Source: CAD feature listing. Evaluate the final solid. Frame: model axes, mm. Face numbers are marked on the shaded views. A direction names the side the tool comes from. Give positions to 0.01 mm unless a question says otherwise; leave off trailing zeros. Order: outer loops, then holes, each group sorted by start corner. A loop starts at its lowest first (then second) coordinate and runs counter-clockwise, first axis right, second up. Notation, with made-up numbers: (65, 34.5) - (106, 34.5) arc R14 ccw to (106, 48.5) - close; hole circle Ø11 at (51, 83). An arc over 180 degrees is marked (long way). Write each question's results on one line, items separated by ' | '. Start each with the question number.
Item 1: Section C-C on y = 1912.5. Output: boundary loops of the cut face in (x, z), and give its area (3 significant figures).
Item 2: Mould query, pull axis X, two halves, no side actions, for the marked faces 1, 2 and 3. Classes: released by +X, released by -X, zero draft, split by the parting line, or undercut.
Item 3: Contact query for flat-ended pins moving along their axis: pin 1 Ø0.9 at (y, z) = (1912, 1) entering from +X; pin 2 Ø1.5 at (y, z) = (1894.5, 1) entering from -X; pin 3 Ø1.5 at (x, z) = (2694.5, 1) entering from +Y. Output: stop coordinate, or through.
Item 4: Set-up query: the marked faces 4, 5 and 6. Return all of +Z, -Z, +X, -X, +Y, -Y with unobstructed straight access to the full face (end or side cutting, diameter ignored); none if empty.
Item 5: Section D-D on z = 0.6. State how many separate pieces and enclosed holes the cut face has, and give its area (3 significant figures).
Item 6: Section A-A on x = 2724.5. Output: boundary loops of the cut face in (y, z), and give its area (3 significant figures).
Item 7: Section B-B on x = 2709.5. Output: boundary loops of the cut face in (y, z), and give its area (3 significant figures).
Item 8: Line query: line 1 along X through (y, z) = (1909, 0.9); line 2 along X through (y, z) = (1897.5, 1); line 3 along X through (y, z) = (1901, 1.65). Output: solid intervals per line, ascending.
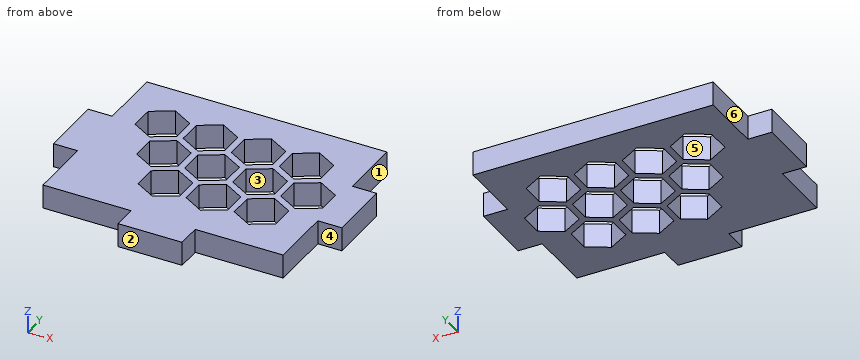
```python
from build123d import *

# Parameters (mm, degrees)
EXTRUDE_1_DEPTH = 3


with BuildPart() as part:
    # 草图1 → 凸台-拉伸1 (new body)
    with BuildSketch(Plane.XY):
        Polygon((2696.149099258, 1909.156494091), (2696.149099258, 1917.111494091), (2707.149099258, 1917.111494091), (2715.149099258, 1917.111494091), (2726.149099258, 1917.111494091), (2726.149099258, 1909.156494091), (2729.149099258, 1909.156494091), (2729.149099258, 1901.156494091), (2726.149099258, 1901.156494091), (2726.149099258, 1893.201494091), (2715.149099258, 1893.201494091), (2715.149099258, 1890.201494091), (2707.149099258, 1890.201494091), (2707.149099258, 1893.201494091), (2696.149099258, 1893.201494091), (2696.149099258, 1901.156494091), (2693.149099258, 1901.156494091), (2693.149099258, 1909.156494091), align=None)
        Polygon((2699.145425292, 1908.906494091), (2701.743501504, 1907.406494091), (2704.341577715, 1908.906494091), (2704.341577715, 1911.906494091), (2701.743501504, 1913.406494091), (2699.145425292, 1911.906494091), align=None, mode=Mode.SUBTRACT)
        Polygon((2705.145425292, 1908.906494091), (2707.743501504, 1907.406494091), (2710.341577715, 1908.906494091), (2710.341577715, 1911.906494091), (2707.743501504, 1913.406494091), (2705.145425292, 1911.906494091), align=None, mode=Mode.SUBTRACT)
        Polygon((2711.145425292, 1908.906494091), (2713.743501504, 1907.406494091), (2716.341577715, 1908.906494091), (2716.341577715, 1911.906494091), (2713.743501504, 1913.406494091), (2711.145425292, 1911.906494091), align=None, mode=Mode.SUBTRACT)
        Polygon((2717.145425292, 1908.906494091), (2719.743501504, 1907.406494091), (2722.341577715, 1908.906494091), (2722.341577715, 1911.906494091), (2719.743501504, 1913.406494091), (2717.145425292, 1911.906494091), align=None, mode=Mode.SUBTRACT)
        Polygon((2702.176514206, 1903.656494091), (2704.774590417, 1902.156494091), (2707.372666628, 1903.656494091), (2707.372666628, 1906.656494091), (2704.774590417, 1908.156494091), (2702.176514206, 1906.656494091), align=None, mode=Mode.SUBTRACT)
        Polygon((2708.176514206, 1903.656494091), (2710.774590417, 1902.156494091), (2713.372666628, 1903.656494091), (2713.372666628, 1906.656494091), (2710.774590417, 1908.156494091), (2708.176514206, 1906.656494091), align=None, mode=Mode.SUBTRACT)
        Polygon((2714.176514206, 1903.656494091), (2716.774590417, 1902.156494091), (2719.372666628, 1903.656494091), (2719.372666628, 1906.656494091), (2716.774590417, 1908.156494091), (2714.176514206, 1906.656494091), align=None, mode=Mode.SUBTRACT)
        Polygon((2720.176514206, 1903.656494091), (2722.774590417, 1902.156494091), (2725.372666628, 1903.656494091), (2725.372666628, 1906.656494091), (2722.774590417, 1908.156494091), (2720.176514206, 1906.656494091), align=None, mode=Mode.SUBTRACT)
        Polygon((2705.207603119, 1898.406494091), (2707.80567933, 1896.906494091), (2710.403755542, 1898.406494091), (2710.403755542, 1901.406494091), (2707.80567933, 1902.906494091), (2705.207603119, 1901.406494091), align=None, mode=Mode.SUBTRACT)
        Polygon((2711.207603119, 1898.406494091), (2713.80567933, 1896.906494091), (2716.403755542, 1898.406494091), (2716.403755542, 1901.406494091), (2713.80567933, 1902.906494091), (2711.207603119, 1901.406494091), align=None, mode=Mode.SUBTRACT)
        Polygon((2717.207603119, 1898.406494091), (2719.80567933, 1896.906494091), (2722.403755542, 1898.406494091), (2722.403755542, 1901.406494091), (2719.80567933, 1902.906494091), (2717.207603119, 1901.406494091), align=None, mode=Mode.SUBTRACT)
    extrude(amount=EXTRUDE_1_DEPTH)


solid = part.part
```
Evaluation:
1) outline: (2696.15, 0) - (2700.17, 0) - (2700.17, 3) - (2696.15, 3) - close; (2703.31, 0) - (2706.17, 0) - (2706.17, 3) - (2703.31, 3) - close; (2709.31, 0) - (2712.17, 0) - (2712.17, 3) - (2709.31, 3) - close; (2715.31, 0) - (2718.17, 0) - (2718.17, 3) - (2715.31, 3) - close; (2721.31, 0) - (2726.15, 0) - (2726.15, 3) - (2721.31, 3) - close | area: 52.3 mm^2
2) face 1: released by +X | face 2: zero draft | face 3: undercut
3) pin 1: stops at x = 2726.15 | pin 2: stops at x = 2696.15 | pin 3: stops at y = 1909.16
4) face 4: +Z, -Z, +X, -Y | face 5: +Z, -Z | face 6: +Z, -Z, -X, +Y
5) separate pieces: 1 | enclosed holes: 11 | area: 532 mm^2
6) outline: (1893.2, 0) - (1903.15, 0) - (1903.15, 3) - (1893.2, 3) - close; (1907.16, 0) - (1917.11, 0) - (1917.11, 3) - (1907.16, 3) - close | area: 59.7 mm^2
7) outline: (1890.2, 0) - (1897.88, 0) - (1897.88, 3) - (1890.2, 3) - close; (1901.93, 0) - (1902.89, 0) - (1902.89, 3) - (1901.93, 3) - close; (1907.42, 0) - (1908.42, 0) - (1908.42, 3) - (1907.42, 3) - close; (1912.39, 0) - (1917.11, 0) - (1917.11, 3) - (1912.39, 3) - close | area: 43.1 mm^2
8) line 1: x = 2693.15 to 2699.15, 2704.34 to 2705.15, 2710.34 to 2711.15, 2716.34 to 2717.15, 2722.34 to 2729.15 | line 2: x = 2696.15 to 2706.78, 2708.83 to 2712.78, 2714.83 to 2718.78, 2720.83 to 2726.15 | line 3: x = 2696.15 to 2705.21, 2710.4 to 2711.21, 2716.4 to 2717.21, 2722.4 to 2726.15
